```python
from build123d import *

# Parameters (mm, degrees)
BOSS_EXTRUDE1_DEPTH      = 14.25
BOSS_EXTRUDE1_DEPTH_BACK = 14.25
CUT_EXTRUDE1_REACH       = 27.192
CUT_EXTRUDE2_REACH       = 25.55
SKETCH3_R                = 1.55


with BuildPart() as part:
    # Sketch1 → Boss-Extrude1 (new, two sides: drawn at the far end of the back side and taken through both)
    with BuildSketch(Plane.XY.offset(-BOSS_EXTRUDE1_DEPTH_BACK)):
        with BuildLine():
            Line((1, 0), (1, 7.75))
            ThreePointArc((1, 7.75), (1.439339828, 8.810660172), (2.5, 9.25))
            Line((2.5, 9.25), (14, 9.25))
            Line((14, 9.25), (16, 9.25))
            Line((16, 9.25), (16, 11.25))
            Line((16, 11.25), (14, 11.25))
            Line((14, 11.25), (2, 11.25))
            ThreePointArc((2, 11.25), (-0.121320344, 10.371320344), (-1, 8.25))
            Line((-1, 8.25), (-1, 0))
            Line((-1, 0), (-1, -2))
            Line((-1, -2), (1, -2))
            Line((1, -2), (1, 0))
        make_face()
    extrude(amount=BOSS_EXTRUDE1_DEPTH + BOSS_EXTRUDE1_DEPTH_BACK)

    # Sketch2 → Cut-Extrude1 (cut, up to next)
    with BuildSketch(Plane(origin=(0, 11.25, 0), x_dir=(1, 0, 0), z_dir=(0, 1, 0)), mode=Mode.PRIVATE) as cut_extrude1_sk1:
        with BuildLine():
            Line((6.248241471, -10.035), (6.248241471, -6.465))
            ThreePointArc((6.248241471, -6.465), (12.28, -8.25), (6.248241471, -10.035))
        make_face()
    cut_extrude1_tool1 = extrude(cut_extrude1_sk1.sketch, amount=-CUT_EXTRUDE1_REACH, mode=Mode.PRIVATE) & part.part
    # Sketch2 → Cut-Extrude1 (cut, up to next)
    with BuildSketch(Plane(origin=(0, 11.25, 0), x_dir=(1, 0, 0), z_dir=(0, 1, 0)), mode=Mode.PRIVATE) as cut_extrude1_sk2:
        with BuildLine():
            Line((6.248241471, 6.465), (6.248241471, 10.035))
            ThreePointArc((6.248241471, 10.035), (12.28, 8.25), (6.248241471, 6.465))
        make_face()
    cut_extrude1_tool2 = extrude(cut_extrude1_sk2.sketch, amount=-CUT_EXTRUDE1_REACH, mode=Mode.PRIVATE) & part.part
    add(cut_extrude1_tool1.solids().sort_by_distance((9.116595, 11.25, 8.25))[0], mode=Mode.SUBTRACT)
    add(cut_extrude1_tool2.solids().sort_by_distance((9.116595, 11.25, -8.25))[0], mode=Mode.SUBTRACT)

    # Sketch3 → Cut-Extrude2 (cut, up to next)
    with BuildSketch(Plane(origin=(1, 0, 0), x_dir=(0, 0, -1), z_dir=(1, 0, 0)), mode=Mode.PRIVATE) as cut_extrude2_sk1:
        with Locations((-7.5, 2.875)):
            Circle(SKETCH3_R)
    cut_extrude2_tool1 = extrude(cut_extrude2_sk1.sketch, amount=-CUT_EXTRUDE2_REACH, mode=Mode.PRIVATE) & part.part
    # Sketch3 → Cut-Extrude2 (cut, up to next)
    with BuildSketch(Plane(origin=(1, 0, 0), x_dir=(0, 0, -1), z_dir=(1, 0, 0)), mode=Mode.PRIVATE) as cut_extrude2_sk2:
        with Locations((7.5, 2.875)):
            Circle(SKETCH3_R)
    cut_extrude2_tool2 = extrude(cut_extrude2_sk2.sketch, amount=-CUT_EXTRUDE2_REACH, mode=Mode.PRIVATE) & part.part
    add(cut_extrude2_tool1.solids().sort_by_distance((1, 2.875, 7.5))[0], mode=Mode.SUBTRACT)
    add(cut_extrude2_tool2.solids().sort_by_distance((1, 2.875, -7.5))[0], mode=Mode.SUBTRACT)


solid = part.part
```
Geometry check sheet. Reference: the model listing, model coordinates, mm. A direction names the side the tool comes from. Give positions to 0.01 mm unless a question says otherwise; leave off trailing zeros. Write each loop counter-clockwise with the first axis right and the second up, starting at its lowest first coordinate (ties: lowest second). Pieces come first, ordered by that corner, then holes. Notation, with made-up numbers: (78, 11) - (90, 11) arc R16 ccw to (90, 24) - close; hole circle Ø11 at (-5.5, -34.75). An arc over 180 degrees is marked (long way). Use a Markdown table: item, result.
Q1. Draft check along Y on faces 1 (the face through (0.014, 1.362, 7.836)), 2 (the face through (12.278, 10.264, 8.132)), 3 (the face through (1.43, 8.8, -0.2)). Enter one of: pulls with the +Y half, pulls with the -Y half, needs draft (parallel to the pull), parting line crosses it, or undercut.
Computed:
| item | result |
|---|---|
| face 1 | undercut |
| face 2 | needs draft |
| face 3 | pulls with the -Y half |
Q2. Section check D-D, the plane y = 9.75. Enter the section's corners in (x, z) (3 decimals), then the cut area to 3 significant figures.
Computed:
| item | result |
|---|---|
| outline | (-0.598, -14.25) - (16, -14.25) - (16, 14.25) - (-0.598, 14.25) - close; hole (6.248, -10.035) arc R3.28 ccw (long way) to (6.248, -6.465) - close; hole (6.248, 6.465) arc R3.28 ccw (long way) to (6.248, 10.035) - close |
| area | 408 mm² |
Q3. Thickness scan on L1, parallel to Z at x = 9, y = 9.7; L2, parallel to Z at x = 0, y = 1.5; L3, parallel to Y at x = 9.5, z = -0.25. Record the ranges inside material, lowest first. Write a range as [from, to].
Computed:
| item | result |
|---|---|
| L1 | z = [-14.25, -11.53], [-4.97, 4.97], [11.53, 14.25] |
| L2 | z = [-14.25, -8.22], [-6.78, 6.78], [8.22, 14.25] |
| L3 | y = [9.25, 11.25] |
Q4. Section check C-C, the plane z = 7.5. Enter the section's corners in (x, y) (3 decimals), then the cut area to 3 significant figures.
Computed:
| item | result |
|---|---|
| outline | (-1, -2) - (1, -2) - (1, 1.325) - (-1, 1.325) - close; (-1, 4.425) - (1, 4.425) - (1, 7.75) arc R1.5 cw to (2.5, 9.25) - (6.248, 9.25) - (6.248, 11.25) - (2, 11.25) arc R3 ccw to (-1, 8.25) - close; (12.193, 9.25) - (16, 9.25) - (16, 11.25) - (12.193, 11.25) - close |
| area | 37.0 mm² |
Q5. Set-up check for faces 4 (the face through (9, 9.25, 0)), 5 (the face through (6.248, 10, 8)), 6 (the face through (0, -2, 0)): record each of +Z, -Z, +X, -X, +Y, -Y from which the full face is reachable in a straight line by a thin tool's end or side.
Computed:
| item | result |
|---|---|
| face 4 | +Z, -Z, +X, -Y |
| face 5 | +Y, -Y |
| face 6 | +Z, -Z, +X, -X, -Y |
Q6. Section check B-B, the plane z = -0.75. Enter the section's corners in (x, y).
Computed:
| item | result |
|---|---|
| outline | (-1, -2) - (1, -2) - (1, 7.75) arc R1.5 cw to (2.5, 9.25) - (16, 9.25) - (16, 11.25) - (2, 11.25) arc R3 ccw to (-1, 8.25) - close |
Q7. Section check A-A, the plane x = 9. Enter the section's corners in (y, z), then the cut area to 3 significant figures.
Computed:
| item | result |
|---|---|
| outline | (9.25, -14.25) - (11.25, -14.25) - (11.25, -11.53) - (9.25, -11.53) - close; (9.25, -4.97) - (11.25, -4.97) - (11.25, 4.97) - (9.25, 4.97) - close; (9.25, 11.53) - (11.25, 11.53) - (11.25, 14.25) - (9.25, 14.25) - close |
| area | 30.8 mm² |
Q8. Go/stop test with flat-tipped pins: P1, Ø6, axis at x = 9, z = 8.25, coming from the -Y side; P2, Ø2, axis at y = 1.5, z = 11, coming from the +X side. Record where each tip stops, or that it passes through.
Computed:
| item | result |
|---|---|
| P1 | stops at y = 9.25 |
| P2 | stops at x = 1 |
